The model under review builds one solid part; all positions refer to its coordinate system, in mm. A direction names the side the tool comes from. Coordinates: 2 decimals unless noted, no trailing zeros. Order: outer loops, then holes, each group sorted by start corner. A loop starts at its lowest first (then second) coordinate and runs counter-clockwise, first axis right, second up. Notation, with made-up numbers: M 21.25,23 L 65.25,23 A28 cw 65.25,41 Z; hole C -21,17 d7. An arc over 180 degrees is marked long. Answer in a Markdown table with one row per item.
from build123d import *

# Parameters (mm, degrees)
F0_R     = 5
F1_DEPTH = 3.5
F2_DEPTH = 5
F4_D     = 3.65
F4_DEPTH = 4
F4_TIP   = 1.0965706297
F5_R     = 0.4


with BuildPart() as f1:
    # F0 (on Top) → F1 (new body)
    with BuildSketch(Plane.XY):
        with BuildLine():
            Line((5.9820292349, 0.4956850747), (7.3584798307, 1.4500946799))
            ThreePointArc((7.3584798307, 1.4500946799), (7.2705019945, 1.8411411536), (7.1617586425, 2.2269290844))
            Line((7.1617586425, 2.2269290844), (5.4969577101, 2.4111892074))
            Line((5.4969577101, 2.4111892074), (6.4889321237, 3.7608190456))
            ThreePointArc((6.4889321237, 3.7608190456), (6.278748587, 4.1021111859), (6.0506321133, 4.4316871538))
            Line((6.0506321133, 4.4316871538), (4.4162055233, 4.0654035761))
            Line((4.4162055233, 4.0654035761), (4.916207935, 5.6640003125))
            ThreePointArc((4.916207935, 5.6640003125), (4.6065953452, 5.9185538205), (4.2838257094, 6.1562031555))
            Line((4.2838257094, 6.1562031555), (2.8568889436, 5.279068386))
            Line((2.8568889436, 5.279068386), (2.8107363336, 6.9533992596))
            ThreePointArc((2.8107363336, 6.9533992596), (2.435246019, 7.0936293128), (2.0528003195, 7.2135990219))
            Line((2.0528003195, 7.2135990219), (0.9879841176, 5.9206642232))
            Line((0.9879841176, 5.9206642232), (0.4006778375, 7.4892895037))
            ThreePointArc((0.4006778375, 7.4892895037), (0, 7.5), (-0.4006778375, 7.4892895037))
            Line((-0.4006778375, 7.4892895037), (-0.9879841176, 5.9206642232))
            Line((-0.9879841176, 5.9206642232), (-2.0528003195, 7.2135990219))
            ThreePointArc((-2.0528003195, 7.2135990219), (-2.435246019, 7.0936293128), (-2.8107363336, 6.9533992596))
            Line((-2.8107363336, 6.9533992596), (-2.8568889436, 5.279068386))
            Line((-2.8568889436, 5.279068386), (-4.2838257094, 6.1562031555))
            ThreePointArc((-4.2838257094, 6.1562031555), (-4.6065953452, 5.9185538205), (-4.916207935, 5.6640003125))
            Line((-4.916207935, 5.6640003125), (-4.4162055233, 4.0654035761))
            Line((-4.4162055233, 4.0654035761), (-6.0506321133, 4.4316871538))
            ThreePointArc((-6.0506321133, 4.4316871538), (-6.278748587, 4.1021111859), (-6.4889321237, 3.7608190456))
            Line((-6.4889321237, 3.7608190456), (-5.4969577101, 2.4111892074))
            Line((-5.4969577101, 2.4111892074), (-7.1617586425, 2.2269290844))
            ThreePointArc((-7.1617586425, 2.2269290844), (-7.2705019945, 1.8411411536), (-7.3584798307, 1.4500946799))
            Line((-7.3584798307, 1.4500946799), (-5.9820292349, 0.4956850747))
            Line((-5.9820292349, 0.4956850747), (-7.4967974966, -0.2191513057))
            ThreePointArc((-7.4967974966, -0.2191513057), (-7.4743836976, -0.619345091), (-7.4306220695, -1.0177699448))
            Line((-7.4306220695, -1.0177699448), (-5.8188550714, -1.4735342273))
            Line((-5.8188550714, -1.4735342273), (-7.0194420172, -2.6414832514))
            ThreePointArc((-7.0194420172, -2.6414832514), (-6.8682999499, -3.0127156849), (-6.697541109, -3.3753434037))
            Line((-6.697541109, -3.3753434037), (-5.025117672, -3.2830732315))
            Line((-5.025117672, -3.2830732315), (-5.7814210773, -4.7775694999))
            ThreePointArc((-5.7814210773, -4.7775694999), (-5.51792933, -5.0796117872), (-5.2386776463, -5.367146031))
            Line((-5.2386776463, -5.367146031), (-3.6868308001, -4.7368403089))
            Line((-3.6868308001, -4.7368403089), (-3.9168934558, -6.3959319615))
            ThreePointArc((-3.9168934558, -6.3959319615), (-3.5696054478, -6.596053134), (-3.2121221742, -6.7773351059))
            Line((-3.2121221742, -6.7773351059), (-1.949018604, -5.6772972392))
            Line((-1.949018604, -5.6772972392), (-1.6279096514, -7.321195952))
            ThreePointArc((-1.6279096514, -7.321195952), (-1.2344594271, -7.3977097755), (-0.8374834233, -7.4530947609))
            Line((-0.8374834233, -7.4530947609), (0, -6.0025309213))
            Line((0, -6.0025309213), (0.8374834233, -7.4530947609))
            ThreePointArc((0.8374834233, -7.4530947609), (1.2344594271, -7.3977097755), (1.6279096514, -7.321195952))
            Line((1.6279096514, -7.321195952), (1.949018604, -5.6772972392))
            Line((1.949018604, -5.6772972392), (3.2121221742, -6.7773351059))
            ThreePointArc((3.2121221742, -6.7773351059), (3.5696054478, -6.596053134), (3.9168934558, -6.3959319615))
            Line((3.9168934558, -6.3959319615), (3.6868308001, -4.7368403089))
            Line((3.6868308001, -4.7368403089), (5.2386776463, -5.367146031))
            ThreePointArc((5.2386776463, -5.367146031), (5.51792933, -5.0796117872), (5.7814210773, -4.7775694999))
            Line((5.7814210773, -4.7775694999), (5.025117672, -3.2830732315))
            Line((5.025117672, -3.2830732315), (6.697541109, -3.3753434037))
            ThreePointArc((6.697541109, -3.3753434037), (6.8682999499, -3.0127156849), (7.0194420172, -2.6414832514))
            Line((7.0194420172, -2.6414832514), (5.8188550714, -1.4735342273))
            Line((5.8188550714, -1.4735342273), (7.4306220695, -1.0177699448))
            ThreePointArc((7.4306220695, -1.0177699448), (7.4743836976, -0.619345091), (7.4967974966, -0.2191513057))
            Line((7.4967974966, -0.2191513057), (5.9820292349, 0.4956850747))
        make_face()
        Circle(F0_R, mode=Mode.SUBTRACT)
    extrude(amount=F1_DEPTH)

    # F0 (on Top) → F2 (join)
    with BuildSketch(Plane.XY):
        Circle(F0_R)
    extrude(amount=F2_DEPTH)

    # F4
    with Locations(Plane.XY.offset(5)):
        with Locations((0, 0)):
            Hole(F4_D / 2, depth=F4_DEPTH)
            with Locations((0, 0, -(F4_DEPTH + F4_TIP / 2))):  # 118° drill point
                Cone(0, F4_D / 2, F4_TIP, mode=Mode.SUBTRACT)

    # F5
    f5_edges = [f1.edges().sort_by_distance(p)[0] for p in [
        (-5, 0, 5),
    ]]
    fillet(f5_edges, radius=F5_R)


solid = f1.part
(1) To check wall thickness, follow line 1 (Y direction, x = 0, z = 3.55) (3 decimals); line 2 (Z direction, x = -6, y = 3.25); line 3 (X direction, y = 6.75, z = 1.4). State the ranges of each line that lie inside material, in increasing order. Write a range as [from, to].
Report:
| item | result |
|---|---|
| line 1 | [-5, -1.825], [1.825, 5] |
| line 2 | [0, 3.5] |
| line 3 | [-2.82, -1.67], [-0.68, 0.68], [1.67, 2.82] |
(2) Take a section at B-B (y = 6.5). Write out the cut boundary in (x, z), then the cut area to 3 significant figures.
Report:
| item | result |
|---|---|
| outline | M -2.82,0 L -1.47,0 L -1.47,3.5 L -2.82,3.5 Z; M -0.77,0 L 0.77,0 L 0.77,3.5 L -0.77,3.5 Z; M 1.47,0 L 2.82,0 L 2.82,3.5 L 1.47,3.5 Z |
| area | 14.9 mm^2 |
(3) The part is to be moulded in two halves that separate along X. For faces 4 (the flat face through (0.413, -6.718, 1.726)), 5 (the flat face through (6.75, 0.133, 1.726)), 6 (the cylindrical face through (0, 7.5, 1.7)), 7 (the flat face through (1.786, -6.511, 1.726)), say which applies: +X half, -X half, draft (parallel to the pull), parting line (faces both ways), or undercut.
Report:
| item | result |
|---|---|
| face 4 | undercut |
| face 5 | +X half |
| face 6 | parting line |
| face 7 | undercut |
(4) Machinability: for faces 1 (the flat face through (-0.69, 6.72, 1.73)), 2 (the flat face through (-1.79, -6.49, 1.73)), 3 (the flat face through (3.803, -5.578, 1.726)), which of the approach directions +Z, -Z, +X, -X, +Y, -Y give a long, thin tool a straight path to every point of the face, cutting with its end or side? Answer none if there is none.
Report:
| item | result |
|---|---|
| face 1 | +Z, -Z, +Y |
| face 2 | +Z, -Z, -Y |
| face 3 | +Z, -Z |
(5) Insertion check: P1, Ø3, axis at y = -2, z = 2.5, coming from the -X side; P2, Ø1, axis at y = -4, z = 2, coming from the +X side; P3, Ø3.5, axis at x = 0, y = 0, coming from the -Z side; P4, Ø1, axis at y = 1, z = 2.5, coming from the -X side. Each pin has a flat end and moves straight along its axis. Give the tip position at first contact, or say it passes through.
Report:
| item | result |
|---|---|
| P1 | x = -7.48 |
| P2 | x = 5.64 |
| P3 | z = 0 |
| P4 | x = -7.36 |
(6) Take a section at A-A (y = 0). Write out the cut boundary in (x, z) (3 decimals).
Report:
| item | result |
|---|---|
| outline | M -7.032,0 L -0.161,0 L -1.825,1 L -1.825,5 L -4.6,5 A0.4 ccw -5,4.6 L -5,3.5 L -7.032,3.5 Z; M 0.161,0 L 7.032,0 L 7.032,3.5 L 5,3.5 L 5,4.6 A0.4 ccw 4.6,5 L 1.825,5 L 1.825,1 Z |
(7) Take a section at C-C (z = 3.9). Write out the cut boundary in (x, y) (3 decimals), then the cut area to 3 significant figures.
Report:
| item | result |
|---|---|
| outline | C 0,0 d10; hole C 0,0 d3.65 |
| area | 68.1 mm^2 |
